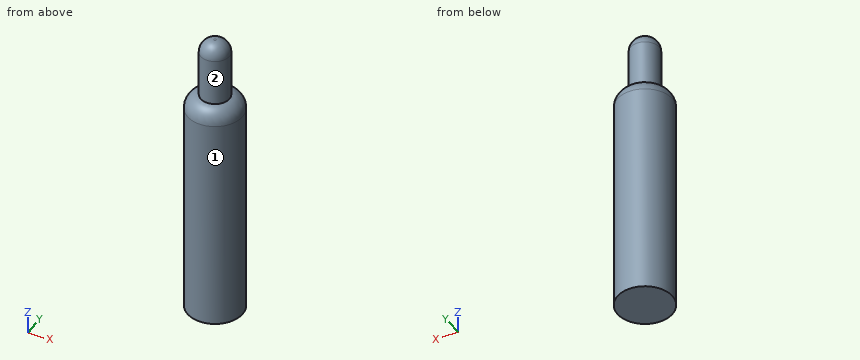
from build123d import *

# Parameters (mm, degrees)
F0_R     = 92.9783177543
F1_DEPTH = 787.4
F2_R     = 48.5104266544
F3_DEPTH = 203.2
F4_R     = 44.45


# Not quite as in the source:
# - a fillet or chamfer that OpenCascade refuses, or shapes differently, is made with other operations: its cross-section is extruded or revolved along the edge and cut away or added


with BuildPart() as f1:
    # F0 (on Top) → F1 (new body)
    with BuildSketch(Plane.XY):
        Circle(F0_R)
    extrude(amount=F1_DEPTH)

    # F2 (on face) → F3 (join)
    with BuildSketch(Plane.XY.offset(787.4)):
        Circle(F2_R)
    extrude(amount=F3_DEPTH)

    # F4
    f4_edges = [f1.edges().sort_by_distance(p)[0] for p in [
        (-48.510427, 0, 990.6),
    ]]
    fillet(f4_edges, radius=F4_R)

    # F5: fillet of radius 50.8 on 1 edges, made by hand

    # F5_s1 → F5_t2 (revolve, cut)
    with BuildSketch(Plane.XZ):
        with BuildLine():
            ThreePointArc((48.5104266544, 787.4), (80.2723535875, 770.6039898535), (92.9783177543, 736.9961866832))
            Line((92.9783177543, 736.9961866832), (92.9783177543, 787.4))
            Line((92.9783177543, 787.4), (48.5104266544, 787.4))
        make_face()
    revolve(axis=Axis((0, 0, 787.4), (0, 0, 1)), mode=Mode.SUBTRACT)


solid = f1.part
Can you work these out from the model? Positions are in its coordinate system, mm. Face numbers are marked on the shaded views. A direction names the side the tool comes from. Round coordinates to 2 decimals unless told otherwise and drop trailing zeros. Loops run counter-clockwise (first coordinate to the right, second up) from the corner with the lowest first, then second, coordinate; pieces in that order, holes last. Notation, with made-up numbers: (50.25, 8) - (97.25, 8) arc R16 ccw to (97.25, 34) - close; hole circle Ø2 at (-13, 17). An arc over 180 degrees is marked (long way). Answer in a Markdown table with one row per item. Add a question column.
Q1. I want a section at B-B on z = 923. List the corners of the cut face in (x, y) for me, and give its area (3 significant figures).
Q2. For pin 1 Ø1.5 at (y, z) = (53, 313.5) entering from +X; pin 2 Ø3 at (y, z) = (33, 859.5) entering from +X; pin 3 Ø6 at (y, z) = (-50.5, 273.5) entering from +X, each with a flat end and sliding along its axis, tell me the tip position at first contact or that it passes through.
Q3. Which directions (+Z, -Z, +X, -X, +Y, -Y) give clear straight access to the entire face, cutting with the end or side of a thin tool? Please do the marked faces 1 and 2.
Q4. I want a section at A-A on z = 269. List the corners of the cut face in (x, y) for me, and give its area (3 significant figures).
Q5. I need wall thicknesses on L1, parallel to Y at x = -1.5, z = 72.5; L2, parallel to Y at x = -3.5, z = 842; L3, parallel to Z at x = 25, y = 68.5. Which ranges of each line are inside material? Lowest first, please.
A:
| question | item | result |
|---|---|---|
| 1 | outline | circle Ø97.02 at (0, 0) |
| 1 | area | 7,390 mm^2 |
| 2 | pin 1 | x = 76.91 |
| 2 | pin 2 | x = 36.89 |
| 2 | pin 3 | x = 79.93 |
| 3 | face 1 | +Z, -Z |
| 3 | face 2 | +Z |
| 4 | outline | circle Ø185.96 at (0, 0) |
| 4 | area | 27,200 mm^2 |
| 5 | L1 | -92.97 to 92.97 |
| 5 | L2 | -48.38 to 48.38 |
| 5 | L3 | 0 to 777.44 |
